Study the drawing (mm; zero at the part's minimum x, y, z) and answer. A direction names the side the tool comes from. Round coordinates to 2 decimals unless told otherwise and drop trailing zeros. Order: outer loops, then holes, each group sorted by start corner. A loop starts at its lowest first (then second) coordinate and runs counter-clockwise, first axis right, second up. Notation, with made-up numbers: (-1, 25) - (50, 25) arc R5 ccw to (50, 31) - close; hole circle Ø3 at (24, 13.5). An arc over 180 degrees is marked (long way). Put each result on its own line as item: value. Start each with the question number.
Q1. Which of the six approach directions +Z, -Z, +X, -X, +Y, -Y give full straight-line access (tool end or side, diameter ignored) to the marked faces 1 and 2?
Q2. Section C-C on z = 20 is taken. Give the vertices of the cut face in (x, y).
Q3. Each of these flat-tipped pins is pushed along its axis until it touches: pin 1 Ø5 at (x, z) = (23.5, 15) entering from +Y; pin 2 Ø2 at (y, z) = (16.5, 24.5) entering from +X. Where does it stop, or does it pass through?
Q4. Section B-B on y = 11 is taken. Give the vertices of the cut face in (x, z).
Q5. Section A-A on x = 15.5 is taken. Give the vertices of the cut face in (y, z).
Q6. Section D-D on z = 8 is taken. Give the vertices of the cut face in (x, y).
Q7. Find the intervals of material crossed by line 1 along Z through (x, y) = (1.7, 11); line 2 along Z through (x, y) = (15.5, 1.5); line 3 along X through (y, z) = (11.75, 25), in increasing order. Write a range as from..to.
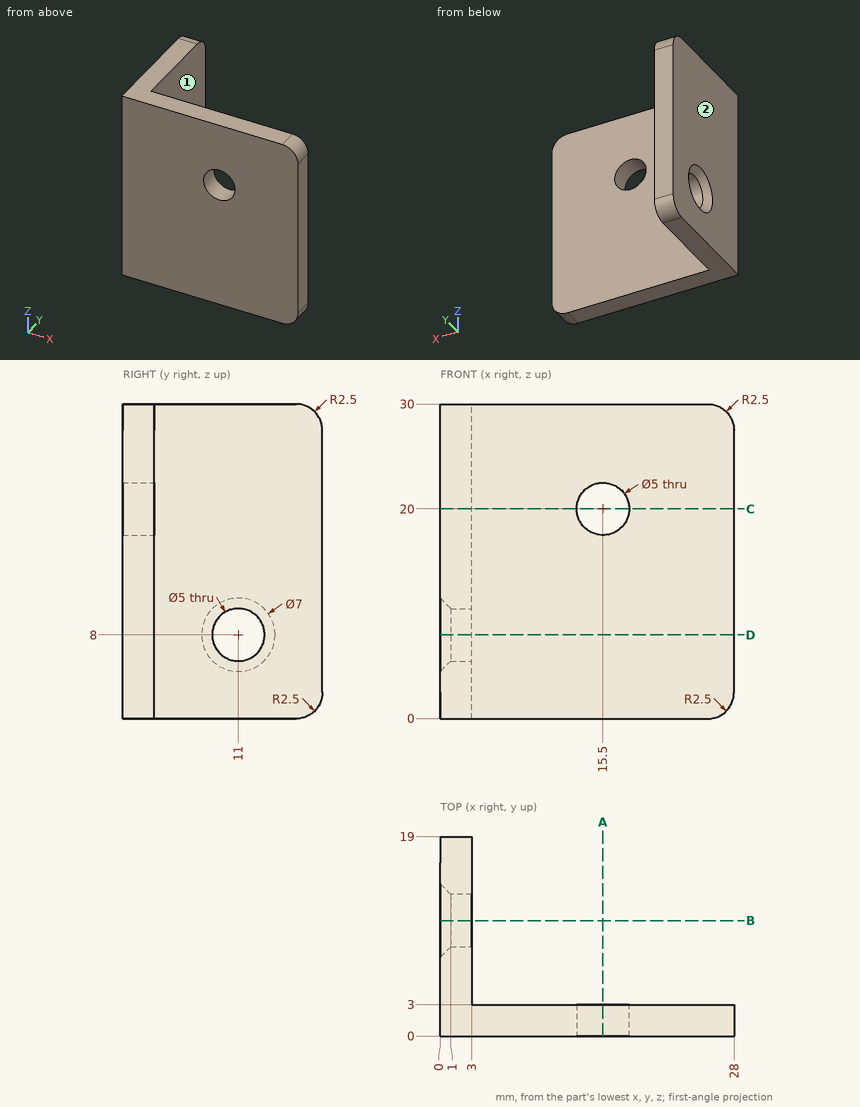
Findings:
1. face 1: +Z, -Z, +X, +Y
1. face 2: +Z, -Z, -X, +Y, -Y
2. outline: (0, 0) - (13, 0) - (13, 3) - (3, 3) - (3, 19) - (0, 19) - close; (18, 0) - (28, 0) - (28, 3) - (18, 3) - close
3. pin 1: y = 3
3. pin 2: x = 3
4. outline: (0, 0) - (3, 0) - (3, 5.5) - (1, 5.5) - (0, 4.5) - close; (0, 11.5) - (1, 10.5) - (3, 10.5) - (3, 30) - (0, 30) - close
5. outline: (0, 0) - (3, 0) - (3, 17.5) - (0, 17.5) - close; (0, 22.5) - (3, 22.5) - (3, 30) - (0, 30) - close
6. outline: (0, 0) - (28, 0) - (28, 3) - (3, 3) - (3, 8.5) - (1, 8.5) - (0, 7.5) - close; (0, 14.5) - (1, 13.5) - (3, 13.5) - (3, 19) - (0, 19) - close
7. line 1: 0..5.5, 10.5..30
7. line 2: 0..17.5, 22.5..30
7. line 3: 0..3
